Can you work these out from the model? Positions are in its coordinate system, mm. Face numbers are marked on the shaded views. A direction names the side the tool comes from. Give positions to 0.01 mm unless a question says otherwise; leave off trailing zeros. Write each loop counter-clockwise with the first axis right and the second up, starting at its lowest first coordinate (ties: lowest second). Pieces come first, ordered by that corner, then holes.
1. On a 3-axis mill with a long thin cutter (end or side, diameter ignored), from which of +Z, -Z, +X, -X, +Y, -Y can I reach the whole of each face in a straight line? I mean the marked faces 1, 2 and 3. Say none if no direction works.
2. Suppose I cut it at B-B (x = 11.5). Please give me the cut outline in (y, z), and give its area (3 significant figures).
3. If I drill on probe 1 along X at (y, z) = (0.7, 8.75); probe 2 along Z at (x, y) = (-1.5, -6.75); probe 3 along Y at (x, z) = (10, -3), over which ranges is the centre line in solid material (lowest first)?
4. I'm going to push flat-ended pins straight in: pin 1 (5 mm diameter, centred on x = 13.5, y = -3, fed in from +Z); pin 2 (12 mm diameter, centred on x = 1.5, z = -8, fed in from -Y); pin 3 (0.5 mm diameter, centred on y = 0.5, z = 3, fed in from -X). Where does each tip first touch, or does it pass through?
5. Suppose I cut it at C-C (y = -6). Please give me the cut outline in (x, z), and give its area (3 significant figures).
6. Suppose I cut it at A-A (z = 8.75). Please give me the cut outline in (x, y).
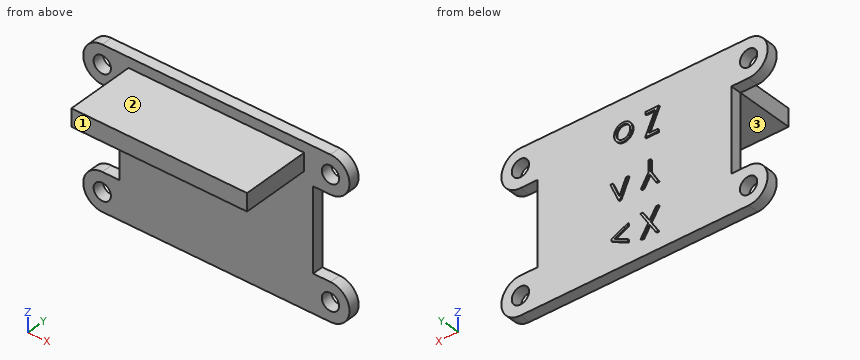
```python
from build123d import *

# Parameters (mm, degrees)
BOSS_EXTRUDE1_DEPTH = 1.6
SKETCH2_R           = 1.25
CUT_EXTRUDE1_DEPTH  = 23.480491543
SKETCH3_W           = 25.4
SKETCH3_H           = 2.54
BOSS_EXTRUDE2_DEPTH = 10
BOSS_EXTRUDE3_DEPTH = 0.2


with BuildPart() as part:
    # Sketch1 → Boss-Extrude1 (new body)
    with BuildSketch(Plane(origin=(0, 0, 0), x_dir=(1, 0, 0), z_dir=(0, 1, 0))):
        with BuildLine():
            Line((-14, 11.5), (-16.5, 11.5))
            ThreePointArc((-16.5, 11.5), (-19.25, 8.75), (-16.5, 6))
            Line((-16.5, 6), (-14, 6))
            Line((-14, 6), (-14, -6))
            Line((-14, -6), (-16.5, -6))
            ThreePointArc((-16.5, -6), (-19.25, -8.75), (-16.5, -11.5))
            Line((-16.5, -11.5), (-14, -11.5))
            Line((-14, -11.5), (14, -11.5))
            Line((14, -11.5), (16.5, -11.5))
            ThreePointArc((16.5, -11.5), (19.25, -8.75), (16.5, -6))
            Line((16.5, -6), (14, -6))
            Line((14, -6), (14, 6))
            Line((14, 6), (16.5, 6))
            ThreePointArc((16.5, 6), (19.25, 8.75), (16.5, 11.5))
            Line((16.5, 11.5), (14, 11.5))
            Line((14, 11.5), (-14, 11.5))
        make_face()
    extrude(amount=BOSS_EXTRUDE1_DEPTH)

    # Sketch2 → Cut-Extrude1 (cut, through all)
    with BuildSketch(Plane(origin=(0, 1.6, 0), x_dir=(1, 0, 0), z_dir=(0, 1, 0))):
        with Locations(Location((-16.5, 8.75, 0), (0, 0, 270))):
            Circle(SKETCH2_R)
        with Locations(Location((16.5, 8.75, 0), (0, 0, 270))):
            Circle(SKETCH2_R)
        with Locations(Location((16.5, -8.75, 0), (0, 0, 270))):
            Circle(SKETCH2_R)
        with Locations(Location((-16.5, -8.75, 0), (0, 0, 270))):
            Circle(SKETCH2_R)
    extrude(amount=-CUT_EXTRUDE1_DEPTH, mode=Mode.SUBTRACT)

    # Sketch3 → Boss-Extrude2 (add)
    with BuildSketch(Plane.XZ):
        with Locations((0, 8.75)):
            Rectangle(SKETCH3_W, SKETCH3_H)
    extrude(amount=BOSS_EXTRUDE2_DEPTH)

    # Sketch4 → Boss-Extrude3 (add)
    # profile 1 of 6: a face of its own
    with BuildSketch(Plane(origin=(0, 1.6, 0), x_dir=(1, 0, 0), z_dir=(0, 1, 0))):
        Polygon((-3.603530873, 9.165262271), (-3.241050905, 9.165262271), (-2.324684719, 7.733571566), (-1.408318533, 9.165262271), (-1.045838565, 9.165262271), (-2.143094174, 7.450318361), (-1.00096677, 5.665262271), (-1.363446738, 5.665262271), (-2.324684719, 7.167065156), (-3.2859227, 5.665262271), (-3.648402668, 5.665262271), (-2.505574142, 7.450318361), align=None)
    # profile 2 of 6: a face of its own
    with BuildSketch(Plane(origin=(0, 1.6, 0), x_dir=(1, 0, 0), z_dir=(0, 1, 0))):
        Polygon((0.771469127, 6.455426534), (2.736012396, 7.392826374), (0.771469127, 8.330226214), (0.771469127, 8.671672528), (3.19454605, 7.515522688), (3.19454605, 7.27013006), (0.771469127, 6.11398022), align=None)
    # profile 3 of 6: a face of its own
    with BuildSketch(Plane(origin=(0, 1.6, 0), x_dir=(1, 0, 0), z_dir=(0, 1, 0))):
        Polygon((-3.62596677, 2.331928938), (-3.26629129, 2.331928938), (-2.346419495, 0.828022688), (-1.427949944, 2.331928938), (-1.068274463, 2.331928938), (-2.190069335, 0.495690957), (-2.190069335, -1.168071062), (-2.504171899, -1.168071062), (-2.504171899, 0.495690957), align=None)
    # profile 4 of 6: a face of its own
    with BuildSketch(Plane(origin=(0, 1.6, 0), x_dir=(1, 0, 0), z_dir=(0, 1, 0))):
        Polygon((1.893263999, 2.331928938), (2.162494768, 2.331928938), (3.329161435, -0.315506959), (2.990519608, -0.315506959), (2.027879383, 1.868487432), (1.065239159, -0.315506959), (0.726597332, -0.315506959), align=None)
    # profile 5 of 6: a face of its own
    with BuildSketch(Plane(origin=(0, 1.6, 0), x_dir=(1, 0, 0), z_dir=(0, 1, 0))):
        Polygon((-3.536223181, -4.860378754), (-3.536223181, -4.501404395), (-1.696479591, -4.501404395), (-3.164628629, -7.642430036), (-1.741351386, -7.642430036), (-1.741351386, -8.001404395), (-3.670838565, -8.001404395), (-2.202689527, -4.860378754), align=None)
    # profile 6 of 6: a face of its own
    with BuildSketch(Plane(origin=(0, 1.6, 0), x_dir=(1, 0, 0), z_dir=(0, 1, 0))):
        with BuildLine():
            add(Edge.make_bspline(
                [(1.468384191, -5.398840293), (1.516375464, -5.399862184), (1.610474622, -5.401865863), (1.748282507, -5.423280828), (1.879827643, -5.456028193), (2.005613835, -5.501299755), (2.124030131, -5.561981705), (2.236801375, -5.634390996), (2.343618384, -5.72017359), (2.407641413, -5.786531658), (2.440138999, -5.820214492)],
                knots=[0, 0, 0, 0, 1.054011418, 2.066658804, 3.057071809, 4.030435133, 4.997543892, 5.974964718, 6.972108034, 8, 8, 8, 8], degree=3))
            add(Edge.make_bspline(
                [(2.440138999, -5.820214492), (2.468120953, -5.852428477), (2.523543333, -5.91623302), (2.594609052, -6.019688632), (2.655830612, -6.126828733), (2.704893573, -6.23907606), (2.743578597, -6.355450731), (2.771044293, -6.476352742), (2.787381228, -6.601515089), (2.789584195, -6.686518927), (2.790699896, -6.729569459)],
                knots=[0, 0, 0, 0, 1.025258237, 2.030674902, 3.01204498, 3.988269485, 4.97094183, 5.956517959, 6.965070386, 8, 8, 8, 8], degree=3))
            add(Edge.make_bspline(
                [(2.790699896, -6.729569459), (2.789718559, -6.772869517), (2.787779391, -6.85843245), (2.769435774, -6.984451816), (2.740904688, -7.106646639), (2.70007285, -7.224505333), (2.647714741, -7.33838816), (2.583824053, -7.447797709), (2.507952436, -7.552949843), (2.421948439, -7.652951681), (2.326896563, -7.745117896), (2.223780415, -7.825446165), (2.114626381, -7.89426769), (1.997983028, -7.949704105), (1.874915541, -7.993413806), (1.745158473, -8.024113822), (1.608913403, -8.042675506), (1.515886181, -8.045059079), (1.468384191, -8.04627619)],
                knots=[0, 0, 0, 0, 0.998656419, 1.973391657, 2.932242238, 3.890759089, 4.846373663, 5.82037756, 6.809684879, 7.83454468, 8.860553229, 9.859544525, 10.845671541, 11.83227036, 12.833544569, 13.85385346, 14.904124723, 16, 16, 16, 16], degree=3))
            add(Edge.make_bspline(
                [(1.468384191, -8.04627619), (1.420649472, -8.045054994), (1.327158612, -8.04266322), (1.19043263, -8.024185937), (1.060443011, -7.993427954), (0.937214412, -7.949560461), (0.820069566, -7.894265918), (0.710283069, -7.825654228), (0.607083153, -7.745094073), (0.512011169, -7.652958136), (0.426012563, -7.55294818), (0.350139555, -7.447798141), (0.286249229, -7.338388048), (0.233891025, -7.224505363), (0.193059212, -7.106646631), (0.164528119, -6.984451818), (0.146184505, -6.85843245), (0.144245336, -6.772869517), (0.143263999, -6.729569459)],
                knots=[0, 0, 0, 0, 1.099876186, 2.154163076, 3.173186993, 4.173200201, 5.163417411, 6.152872554, 7.150605724, 8.17532212, 9.198891216, 10.186952605, 11.159729845, 12.11414092, 13.071450619, 14.029093627, 15.002601286, 16, 16, 16, 16], degree=3))
            add(Edge.make_bspline(
                [(0.143263999, -6.729569459), (0.144387309, -6.686752914), (0.146611271, -6.601983511), (0.16293178, -6.477056451), (0.190290336, -6.356359061), (0.229021733, -6.240433585), (0.278536924, -6.128678149), (0.338898211, -6.021273318), (0.410688844, -5.918285518), (0.465890796, -5.854563438), (0.493824896, -5.822317857)],
                knots=[0, 0, 0, 0, 1.031353054, 2.041901799, 3.029428768, 4.008703097, 4.981709435, 5.96992636, 6.972712378, 8, 8, 8, 8], degree=3))
            add(Edge.make_bspline(
                [(0.493824896, -5.822317857), (0.526273487, -5.788342918), (0.590089351, -5.721525221), (0.697438079, -5.635992697), (0.8099319, -5.562076623), (0.929656826, -5.502600408), (1.055339684, -5.45576189), (1.187558927, -5.423196375), (1.325834442, -5.40194302), (1.420394063, -5.399884842), (1.468384191, -5.398840293)],
                knots=[0, 0, 0, 0, 1.027980169, 2.021703884, 2.998553061, 3.971491411, 4.943284454, 5.930300938, 6.949603206, 8, 8, 8, 8], degree=3))
        make_face()
        with BuildLine():
            add(Edge.make_bspline(
                [(1.466981948, -5.712942857), (1.433044336, -5.713907449), (1.366045208, -5.715811731), (1.267425623, -5.730295636), (1.172485469, -5.75324314), (1.081044625, -5.785847196), (0.993411452, -5.827946095), (0.90950205, -5.879654455), (0.82906961, -5.940287412), (0.753687547, -6.009750083), (0.684505235, -6.085629078), (0.624027258, -6.166477437), (0.572602152, -6.250983783), (0.529761993, -6.339235994), (0.497854805, -6.432128408), (0.474681782, -6.528609039), (0.460211542, -6.628874456), (0.458325163, -6.697035474), (0.457366563, -6.731672825)],
                knots=[0, 0, 0, 0, 1.021534396, 2.016698045, 2.994645724, 3.958388632, 4.93408049, 5.916473867, 6.921342795, 7.962252576, 8.998418191, 10.008913653, 10.997312074, 11.973003931, 12.956656626, 13.948281152, 14.957379055, 16, 16, 16, 16], degree=3))
            add(Edge.make_bspline(
                [(0.457366563, -6.731672825), (0.458973387, -6.776424852), (0.462162631, -6.865249258), (0.488097867, -6.99606038), (0.531484147, -7.121642232), (0.590071427, -7.241258618), (0.663477646, -7.351930896), (0.749964712, -7.450602381), (0.848604413, -7.535788192), (0.958220913, -7.606469038), (1.076575231, -7.662628793), (1.201831552, -7.702427769), (1.332472246, -7.728299462), (1.421752977, -7.730870936), (1.466981948, -7.732173626)],
                knots=[0, 0, 0, 0, 1.016792936, 2.018143844, 3.017858371, 4.030088057, 5.03801393, 6.028138512, 7.003788237, 7.991172063, 8.984598303, 9.972568034, 10.972917682, 12, 12, 12, 12], degree=3))
            add(Edge.make_bspline(
                [(1.466981948, -7.732173626), (1.512208316, -7.730863346), (1.601483912, -7.728276889), (1.731943089, -7.702558069), (1.856857061, -7.662454409), (1.975088449, -7.606532199), (2.084655052, -7.535519784), (2.184004173, -7.451083407), (2.269752785, -7.351669556), (2.343086389, -7.241112027), (2.402633132, -7.121827675), (2.445816334, -6.996037202), (2.47181392, -6.86525516), (2.474994749, -6.77642683), (2.476597332, -6.731672825)],
                knots=[0, 0, 0, 0, 1.02726834, 2.027799167, 3.010890988, 4.004497153, 4.992059811, 5.971914811, 6.958719428, 7.966827853, 8.981595046, 9.981490638, 10.983022906, 12, 12, 12, 12], degree=3))
            add(Edge.make_bspline(
                [(2.476597332, -6.731672825), (2.475639062, -6.697035267), (2.473753333, -6.628873841), (2.459278369, -6.528611388), (2.436122829, -6.432119791), (2.404151212, -6.339267788), (2.361497198, -6.250755284), (2.309080405, -6.166725557), (2.248849379, -6.085349011), (2.178832258, -6.00999537), (2.103528881, -5.940260333), (2.023063842, -5.879630944), (1.939278864, -5.828173348), (1.851900281, -5.785487108), (1.760447714, -5.753539767), (1.665640584, -5.730163136), (1.567441774, -5.715872939), (1.500682731, -5.713925798), (1.466981948, -5.712942857)],
                knots=[0, 0, 0, 0, 1.042956736, 2.052379634, 3.044323526, 4.02829302, 5.004299113, 5.996692471, 7.007513377, 8.048758398, 9.090003419, 10.095195979, 11.07790575, 12.047570684, 13.018257071, 13.989683339, 14.985167495, 16, 16, 16, 16], degree=3))
        make_face(mode=Mode.SUBTRACT)
    extrude(amount=BOSS_EXTRUDE3_DEPTH)


solid = part.part
```
Checks:
1. face 1: +Z, -Z, +X, -X, -Y
1. face 2: +Z, +X, -X, -Y
1. face 3: -Z, +X, -X, -Y
2. outline: (-10, 7.48) - (0, 7.48) - (0, -11.5) - (1.6, -11.5) - (1.6, 11.5) - (0, 11.5) - (0, 10.02) - (-10, 10.02) - close
2. area: 62.2 mm2
3. probe 1: x = -19.25 to -17.75, -15.25 to 15.25, 17.75 to 19.25
3. probe 2: z = 7.48 to 10.02
3. probe 3: y = 0 to 1.6
4. pin 1: stops at z = 10.02
4. pin 2: stops at y = 0
4. pin 3: stops at x = -14
5. outline: (-12.7, 7.48) - (12.7, 7.48) - (12.7, 10.02) - (-12.7, 10.02) - close
5. area: 64.5 mm2
6. outline: (-19.25, 0) - (-17.75, 0) - (-17.75, 1.6) - (-19.25, 1.6) - close; (-15.25, 0) - (-12.7, 0) - (-12.7, -10) - (12.7, -10) - (12.7, 0) - (15.25, 0) - (15.25, 1.6) - (-15.25, 1.6) - close; (17.75, 0) - (19.25, 0) - (19.25, 1.6) - (17.75, 1.6) - close
